Check sheet for the modelled part. Datum: model origin and axes. Units: mm. A direction names the side the tool comes from. Give positions to 0.01 mm unless a question says otherwise; leave off trailing zeros. Order: outer loops, then holes, each group sorted by start corner. A loop starts at its lowest first (then second) coordinate and runs counter-clockwise, first axis right, second up. Notation, with made-up numbers: (-9.5, 27.5) -> (5.5, 27.5) arc R21 ccw to (5.5, 32.5) -> close; hole circle Ø10 at (-37, -32.75). An arc over 180 degrees is marked (long way). One line per question, with ' | ' between items.
```python
from build123d import *

# Parameters (mm, degrees)
SKETCH2_R       = 27.4
EXTRUDE1_DEPTH  = 3
EXTRUDE2_DEPTH  = 3
SKETCH5_R       = 24.971147558
SKETCH5_R_2     = 24.571147558
EXTRUDE3_DEPTH  = 1.5
EXTRUDE4_DEPTH  = 1.5
EXTRUDE11_DEPTH = 3.8
EXTRUDE12_DEPTH = 1.5
FILLET1_R       = 0.5


with BuildPart() as part:
    # Sketch2 → Extrude1 (new body)
    with BuildSketch(Plane.XY):
        Circle(SKETCH2_R)
        with BuildLine():
            Line((-4, 23.055585007), (4, 23.055585007))
            ThreePointArc((4, 23.055585007), (16.54629868, 16.54629868), (23.055585007, 4))
            Line((23.055585007, 4), (23.055585007, -4))
            ThreePointArc((23.055585007, -4), (16.54629868, -16.54629868), (4, -23.055585007))
            Line((4, -23.055585007), (-4, -23.055585007))
            ThreePointArc((-4, -23.055585007), (-16.54629868, -16.54629868), (-23.055585007, -4))
            Line((-23.055585007, -4), (-23.055585007, 4))
            ThreePointArc((-23.055585007, 4), (-16.54629868, 16.54629868), (-4, 23.055585007))
        make_face(mode=Mode.SUBTRACT)
    extrude(amount=EXTRUDE1_DEPTH)

    # Sketch3 → Extrude2 (cut)
    with BuildSketch(Plane.XY.offset(3)):
        with BuildLine():
            Line((-1.893881028, 25.871147558), (1.893881028, 25.871147558))
            ThreePointArc((1.893881028, 25.871147558), (2.710560642, 25.796258258), (3.5, 25.574088282))
            Line((3.5, 25.574088282), (3.5, 23.671147558))
            Line((3.5, 23.671147558), (-3.5, 23.671147558))
            Line((-3.5, 23.671147558), (-3.5, 25.574088282))
            ThreePointArc((-3.5, 25.574088282), (-2.710560642, 25.796258258), (-1.893881028, 25.871147558))
        make_face()
        with BuildLine():
            Line((23.671147558, -3.5), (23.671147558, 3.5))
            Line((23.671147558, 3.5), (25.574088282, 3.5))
            ThreePointArc((25.574088282, 3.5), (25.796258258, 2.710560642), (25.871147558, 1.893881028))
            Line((25.871147558, 1.893881028), (25.871147558, -1.893881028))
            ThreePointArc((25.871147558, -1.893881028), (25.796258258, -2.710560642), (25.574088282, -3.5))
            Line((25.574088282, -3.5), (23.671147558, -3.5))
        make_face()
        with BuildLine():
            Line((-3.5, -23.671147558), (3.5, -23.671147558))
            Line((3.5, -23.671147558), (3.5, -25.574088282))
            ThreePointArc((3.5, -25.574088282), (2.710560642, -25.796258258), (1.893881028, -25.871147558))
            Line((1.893881028, -25.871147558), (-1.893881028, -25.871147558))
            ThreePointArc((-1.893881028, -25.871147558), (-2.710560642, -25.796258258), (-3.5, -25.574088282))
            Line((-3.5, -25.574088282), (-3.5, -23.671147558))
        make_face()
        with BuildLine():
            Line((-23.671147558, 3.5), (-23.671147558, -3.5))
            Line((-23.671147558, -3.5), (-25.574088282, -3.5))
            ThreePointArc((-25.574088282, -3.5), (-25.796258258, -2.710560642), (-25.871147558, -1.893881028))
            Line((-25.871147558, -1.893881028), (-25.871147558, 1.893881028))
            ThreePointArc((-25.871147558, 1.893881028), (-25.796258258, 2.710560642), (-25.574088282, 3.5))
            Line((-25.574088282, 3.5), (-23.671147558, 3.5))
        make_face()
    extrude(amount=-EXTRUDE2_DEPTH, mode=Mode.SUBTRACT)

    # Sketch5 → Extrude3 (cut)
    with BuildSketch(Plane.XY.offset(3)):
        Circle(SKETCH5_R)
        Circle(SKETCH5_R_2, mode=Mode.SUBTRACT)
    extrude(amount=-EXTRUDE3_DEPTH, mode=Mode.SUBTRACT)

    # Sketch6 → Extrude4 (cut)
    with BuildSketch(Plane.XY.offset(3)):
        Polygon((-19.691237457, 16.862810332), (-18.277023894, 15.448596769), (-15.448596769, 18.277023894), (-16.862810332, 19.691237457), align=None)
        Polygon((16.862810332, 19.691237457), (19.691237457, 16.862810332), (18.277023894, 15.448596769), (15.448596769, 18.277023894), align=None)
        Polygon((-19.691237457, -16.862810332), (-18.277023894, -15.448596769), (-15.448596769, -18.277023894), (-16.862810332, -19.691237457), align=None)
        Polygon((6.912025, -24.986458638), (6.231672227, -23.105735345), (9.993118813, -21.745029799), (10.673471586, -23.625753092), align=None)
        Polygon((24.986458638, -6.912025), (23.105735345, -6.231672227), (21.745029799, -9.993118813), (23.625753092, -10.673471586), align=None)
    extrude(amount=-EXTRUDE4_DEPTH, mode=Mode.SUBTRACT)

    # Sketch13 → Extrude11 (cut)
    with BuildSketch(Plane.XY.offset(3)):
        Polygon((19.975766569, -17.642314191), (18.785405345, -16.451952967), (17.936646698, -17.373396778), (17.373396778, -17.936646698), (16.451952967, -18.785405345), (17.642314191, -19.975766569), (19.180190393, -21.513642771), (21.513642771, -19.180190393), align=None)
    extrude(amount=-EXTRUDE11_DEPTH, mode=Mode.SUBTRACT)

    # Sketch14 → Extrude12 (cut)
    with BuildSketch(Plane.XY.offset(3)):
        with BuildLine():
            Line((10.673471586, -23.625753092), (10.279766704, -22.537420726))
            Line((10.279766704, -22.537420726), (9.993118813, -21.745029799))
            ThreePointArc((9.993118813, -21.745029799), (12.986268088, -20.101382682), (15.715013126, -18.048465504))
            ThreePointArc((15.715013126, -18.048465504), (16.922008518, -16.922008518), (18.048465504, -15.715013126))
            ThreePointArc((18.048465504, -15.715013126), (20.101382682, -12.986268088), (21.745029799, -9.993118813))
            Line((21.745029799, -9.993118813), (22.537420726, -10.279766704))
            Line((22.537420726, -10.279766704), (23.625753092, -10.673471586))
            ThreePointArc((23.625753092, -10.673471586), (21.783851689, -14.055710955), (19.461215863, -17.127763485))
            Line((19.461215863, -17.127763485), (17.127763485, -19.461215863))
            ThreePointArc((17.127763485, -19.461215863), (14.055710955, -21.783851689), (10.673471586, -23.625753092))
        make_face()
    extrude(amount=-EXTRUDE12_DEPTH, mode=Mode.SUBTRACT)

    # Fillet1
    fillet1_edges = [part.edges().sort_by_distance(p)[0] for p in [
        (20.506290558, -18.17283818, 1.5),
        (18.17283818, -20.506290558, 1.5),
        (17.127763485, -19.461215863, 2.25),
        (19.461215863, -17.127763485, 2.25),
    ]]
    fillet(fillet1_edges, radius=FILLET1_R)


solid = part.part
```
Q1. Thickness scan on line 1 (Y direction, x = 1.5, z = 0.65); line 2 (Y direction, x = 7, z = 2.6); line 3 (X direction, y = 12.5, z = 2.6). Record the ranges inside material, lowest first.
Result sheet:
line 1: y = -27.36 to -25.87, -23.67 to -23.06, 23.06 to 23.67, 25.87 to 27.36 | line 2: y = -26.49 to -24.95, -22.83 to -22.33, 22.33 to 23.55, 23.97 to 26.49 | line 3: x = -24.38 to -21.62, -21.15 to -19.78, 19.78 to 21.15, 21.62 to 24.38
Q2. Section check B-B (z = 2.4). Count the separate pieces of the cut face and the enclosed holes in it, and give its area (3 significant figures).
Result sheet:
separate pieces: 2 | enclosed holes: 1 | area: 469 mm2
Q3. Depth check by flat-ended pin: pin 1 Ø1.5 at (x, z) = (17, 1.5) entering from +Y; pin 2 Ø0.6 at (x, z) = (24.5, 1) entering from +Y; pin 3 Ø0.6 at (y, z) = (-25, 2) entering from +X; pin 4 Ø8 at (x, y) = (15.5, -2) entering from +Z. Enter the tip coordinate at first touch or a pass-through.
Result sheet:
pin 1: stops at y = 22.06 | pin 2: stops at y = 12.85 | pin 3: stops at x = 11.86 | pin 4: passes through
Q4. Access from +Z, -Z, +X, -X, +Y, -Y to the whole of each face (thin tool, end or side, straight path). Record for faces 1 (the face through (18.257, 18.297, 2.26)), 2 (the face through (0, -23.056, 1)).
Result sheet:
face 1: +Z | face 2: +Z, -Z
Q5. Mould release check, pull along X, two halves, no side actions. Record for faces 3 (the face through (-25.8, -2.7, 1.5)), 4 (the face through (-25, -3.5, 2)): pulls with the +X half, pulls with the -X half, needs draft (parallel to the pull), parting line crosses it, or undercut.
Result sheet:
face 3: undercut | face 4: undercut
Q6. Section check A-A (x = 0). Enter the section's corners in (y, z), and give its area (3 significant figures).
Result sheet:
outline: (-27.4, 0) -> (-25.87, 0) -> (-25.87, 3) -> (-27.4, 3) -> close; (-23.67, 0) -> (-23.06, 0) -> (-23.06, 3) -> (-23.67, 3) -> close; (23.06, 0) -> (23.67, 0) -> (23.67, 3) -> (23.06, 3) -> close; (25.87, 0) -> (27.4, 0) -> (27.4, 3) -> (25.87, 3) -> close | area: 12.9 mm2
Q7. Section check C-C (y = 13). Enter the section's corners in (x, z).
Result sheet:
outline: (-24.12, 0) -> (-19.46, 0) -> (-19.46, 3) -> (-20.85, 3) -> (-20.85, 1.5) -> (-21.32, 1.5) -> (-21.32, 3) -> (-24.12, 3) -> close; (19.46, 0) -> (24.12, 0) -> (24.12, 3) -> (21.32, 3) -> (21.32, 1.5) -> (20.85, 1.5) -> (20.85, 3) -> (19.46, 3) -> close
